```python
from build123d import *

# Parameters (mm, degrees)
MOUNT_DEPTH                  = 17.5
F_1_4_ANTENNA_HOLES_D        = 6.7564
SKETCH6_R                    = 1.65
M3_STANDOFF_HOLES_DEPTH      = 15
M3_STANDOFF_HOLES_DEPTH_BACK = 3
INSIDE_FILLET_R              = 1
EXTERNAL_FILLETS_R           = 0.4


with BuildPart() as part:
    # Sketch1 → Mount (new body, symmetric)
    with BuildSketch(Plane(origin=(0, 0, 0), x_dir=(0, 0, -1), z_dir=(1, 0, 0))):
        Polygon((-2, 16), (0, 16), (0, 0), (-16, 0), (-16, 2), (-2, 2), align=None)
    extrude(amount=MOUNT_DEPTH, both=True)

    # 1/4" Antenna Holes (through all)
    with Locations(Plane.XY.offset(2)):
        with Locations((-8.75, 9), (8.75, 9)):
            Hole(F_1_4_ANTENNA_HOLES_D / 2)

    # Sketch6 → M3 Standoff Holes (cut, two sides)
    with BuildSketch(Plane(origin=(0, 2, 0), x_dir=(1, 0, 0), z_dir=(0, 1, 0))) as m3_standoff_holes_sk:
        with Locations((-7.5, -9)):
            Circle(SKETCH6_R)
        with Locations((7.5, -9)):
            Circle(SKETCH6_R)
    extrude(amount=M3_STANDOFF_HOLES_DEPTH, mode=Mode.SUBTRACT)
    extrude(m3_standoff_holes_sk.sketch, amount=-M3_STANDOFF_HOLES_DEPTH_BACK, mode=Mode.SUBTRACT)

    # Inside Fillet
    inside_fillet_edges = [part.edges().sort_by_distance(p)[0] for p in [
        (0, 2, 2),
    ]]
    fillet(inside_fillet_edges, radius=INSIDE_FILLET_R)

    # External Fillets
    external_fillets_edges = [part.edges().sort_by_distance(p)[0] for p in [
        (0, 16, 2),
        (0, 16, 0),
        (0, 0, 0),
        (0, 0, 16),
        (0, 2, 16),
        (17.5, 1, 16),
        (17.5, 0, 8),
        (17.5, 8, 0),
        (12.1282, 9, 0),
        (17.5, 16, 1),
        (-5.3718, 9, 0),
        (-17.5, 2, 9.5),
        (17.5, 2, 9.5),
        (-17.5, 2.292893219, 2.292893219),
        (17.5, 2.292893219, 2.292893219),
        (17.5, 9.5, 2),
        (-17.5, 16, 1),
        (-17.5, 8, 0),
        (-17.5, 0, 8),
        (-17.5, 1, 16),
        (-17.5, 9.5, 2),
    ]]
    fillet(external_fillets_edges, radius=EXTERNAL_FILLETS_R)


solid = part.part
```
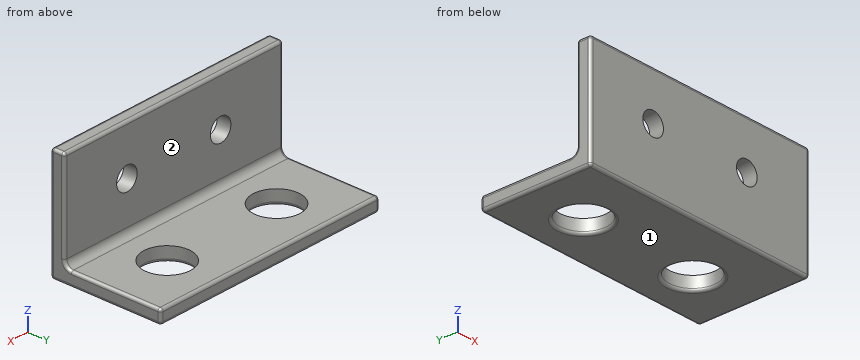
Design review of the part built by this model. Coordinates are the model's own, in mm. Face numbers are marked on the shaded views. A direction names the side the tool comes from. Round coordinates to 2 decimals unless told otherwise and drop trailing zeros. Write each loop counter-clockwise with the first axis right and the second up, starting at its lowest first coordinate (ties: lowest second). Pieces come first, ordered by that corner, then holes. Notation, with made-up numbers: (69.25, -2.75) -> (125.25, -2.75) arc R37 cw to (125.25, 33.25) -> close; hole circle Ø3 at (48.5, 2). An arc over 180 degrees is marked (long way). Write item = value, one per line. Start each with the question number.
1) Take a section at B-B, the plane y = 9. State the section outline as (x, z) points, plus the area to 3 significant figures.
2) Clearance check with flat-ended pins moving along their axes: pin 1 (9 mm diameter, centred on x = 8.75, y = 9, fed in from +Z); pin 2 (1 mm diameter, centred on y = 9.5, z = 4, fed in from -X); pin 3 (1 mm diameter, centred on x = 4, y = 9, fed in from -Z); pin 4 (6.5 mm diameter, centred on x = -1, z = 10.5, fed in from +Y). State where each tip first meets the part, or that it passes through.
3) Wall thickness on probe 1 along X at (y, z) = (1.4, 9); probe 2 along Z at (x, y) = (-7.5, 1.6); probe 3 along Y at (x, z) = (-8.75, 1.25): over which ranges is each line inside the solid? List them lowest first. Write a range as from..to.
4) Tool access review of the marked faces 1 and 2: name each direction out of +Z, -Z, +X, -X, +Y, -Y from which nothing blocks a thin tool from reaching the whole face with its end or side.
5) Take a section at A-A, the plane z = 9. State the section outline as (x, y) points.
6) Take a section at D-D, the plane y = 13.75. State the section outline as (x, z) points.
7) Take a section at C-C, the plane x = -13. State the section outline as (y, z) points.
Results list:
q1.outline = (-17.5, 0.4) arc R0.4 ccw to (-17.1, 0) -> (-12.53, 0) arc R0.4 ccw to (-12.13, 0.4) -> (-12.13, 2) -> (-17.1, 2) arc R0.4 ccw to (-17.5, 1.6) -> close; (-5.37, 0.4) arc R0.4 ccw to (-4.97, 0) -> (4.97, 0) arc R0.4 ccw to (5.37, 0.4) -> (5.37, 2) -> (-5.37, 2) -> close; (12.13, 0.4) arc R0.4 ccw to (12.53, 0) -> (17.1, 0) arc R0.4 ccw to (17.5, 0.4) -> (17.5, 1.6) arc R0.4 ccw to (17.1, 2) -> (12.13, 2) -> close
q1.area = 42.7 mm²
q2.pin_1 = 2
q2.pin_2 = through
q2.pin_3 = 0
q2.pin_4 = 2
q3.probe_1 = -17.5..-9.15, -5.85..5.85, 9.15..17.5
q3.probe_2 = 0..7.35, 10.65..16
q3.probe_3 = 0..5.62, 12.38..16
q4.face_1 = -Z, +X, -X, +Y, -Y
q4.face_2 = +Z, +X, -X, +Y
q5.outline = (-17.5, 0.4) arc R0.4 ccw to (-17.1, 0) -> (-9.15, 0) -> (-9.15, 2) -> (-17.1, 2) arc R0.4 ccw to (-17.5, 1.6) -> close; (-5.85, 0) -> (5.85, 0) -> (5.85, 2) -> (-5.85, 2) -> close; (9.15, 0) -> (17.1, 0) arc R0.4 ccw to (17.5, 0.4) -> (17.5, 1.6) arc R0.4 ccw to (17.1, 2) -> (9.15, 2) -> close
q6.outline = (-17.5, 0.4) arc R0.4 ccw to (-17.1, 0) -> (17.1, 0) arc R0.4 ccw to (17.5, 0.4) -> (17.5, 1.6) arc R0.4 ccw to (17.1, 2) -> (-17.1, 2) arc R0.4 ccw to (-17.5, 1.6) -> close
q7.outline = (0, 0.4) arc R0.4 ccw to (0.4, 0) -> (15.6, 0) arc R0.4 ccw to (16, 0.4) -> (16, 1.6) arc R0.4 ccw to (15.6, 2) -> (3, 2) arc R1 cw to (2, 3) -> (2, 15.6) arc R0.4 ccw to (1.6, 16) -> (0.4, 16) arc R0.4 ccw to (0, 15.6) -> close
